Can you work these out from the model? Positions are in its coordinate system, mm. Give positions to 0.01 mm unless a question says otherwise; leave off trailing zeros. Loops run counter-clockwise (first coordinate to the right, second up) from the corner with the lowest first, then second, coordinate; pieces in that order, holes last. Notation, with made-up numbers: (1, 78) -> (53, 78) arc R22 cw to (53, 98) -> close; hole circle Ø2 at (-18, 10). An arc over 180 degrees is marked (long way). Use CSV: the item, a comma, the result in double quotes.
from build123d import *

# Parameters (mm, degrees)
F1_DEPTH = 400
F3_DEPTH = 25


with BuildPart() as f1:
    # F0 (on Front) → F1 (new body)
    with BuildSketch(Plane.XZ):
        Polygon((-225.0889671236, 36.5147186258), (78.9826564552, 340.5863422045), (65.5983955954, 344.1726440932), (-233.5742484978, 45), align=None)
    extrude(amount=F1_DEPTH)

    # F2 (on face) → F3 (cut)
    with BuildSketch(Plane(origin=(-130.8018428747, 0, 130.8018428747), x_dir=(0, 1, 0), z_dir=(0.7071067812, 0, -0.7071067812))):
        with BuildLine():
            ThreePointArc((-320, 81.668977129), (-200, -38.331022871), (-80, 81.668977129))
            Line((-80, 81.668977129), (-320, 81.668977129))
        make_face()
        with BuildLine():
            Line((-320, 81.668977129), (-80, 81.668977129))
            ThreePointArc((-80, 81.668977129), (-200, 201.668977129), (-320, 81.668977129))
        make_face()
    extrude(amount=-F3_DEPTH, mode=Mode.SUBTRACT)


solid = f1.part
(1) If we section it at D-D, the plane z = 63: Write out the boundary of the cut face in (x, y), then the cut area to 3 significant figures.
Answer sheet:
outline,"(-215.57, -400) -> (-198.6, -400) -> (-198.6, 0) -> (-215.57, 0) -> close"
area,"6,790 mm2"
(2) If we section it at C-C, the plane y = -205: Write out the boundary of the cut face in (x, z).
Answer sheet:
outline,"(-233.57, 45) -> (-225.09, 36.51) -> (-157.83, 103.77) -> (-166.32, 112.26) -> close; (3.24, 281.81) -> (11.73, 273.33) -> (78.98, 340.59) -> (65.6, 344.17) -> close"
(3) We'd pull the mould along Y, two halves only. Please class faces 1 (the face through (-160.071, -226.014, 109.899)), 2 (the face through (-66, -400, 202)), 3 (the face through (-66, 0, 202)): released by +Y, released by -Y, zero draft, split by the parting line, or undercut.
Answer sheet:
face 1,"undercut"
face 2,"released by -Y"
face 3,"released by +Y"
(4) Will these pins go through, and if not, where does the flat tip stop? pin 1 Ø10 at (y, z) = (-322, 148.5) entering from -X; pin 2 Ø1.5 at (y, z) = (-50, 247.5) entering from +X; pin 3 Ø3 at (x, y) = (-1.5, -259.5) entering from -Z; pin 4 Ø1.5 at (x, z) = (-52.5, 207.5) entering from +Y.
Answer sheet:
pin 1,"stops at x = -135.07"
pin 2,"stops at x = -13.35"
pin 3,"stops at z = 262.44"
pin 4,"passes through"
(5) If I drill on L1, parallel to X at y = -347, z = 241; L2, parallel to Z at x = -209, y = -145; L3, parallel to X at y = -236.5, z = 57, over which ranges is the centre line in solid material (lowest first)? Write a range as from..to.
Answer sheet:
L1,"x = -37.57..-20.6"
L2,"z = 52.6..69.57"
L3,"x = -221.57..-204.6"
(6) If we section it at A-A, the plane y = -93: Write out the boundary of the cut face in (x, z), then the cut area to 3 significant figures.
Answer sheet:
outline,"(-233.57, 45) -> (-225.09, 36.51) -> (-111.47, 150.14) -> (-119.95, 158.62) -> close; (-43.13, 235.45) -> (-34.64, 226.96) -> (78.98, 340.59) -> (65.6, 344.17) -> close"
area,"3,810 mm2"
(7) If we section it at B-B, the plane y = -365.5: Write out the boundary of the cut face in (x, z), then the cut area to 3 significant figures.
Answer sheet:
outline,"(-233.57, 45) -> (-225.09, 36.51) -> (78.98, 340.59) -> (65.6, 344.17) -> close"
area,"5,120 mm2"
